Source: CAD feature listing. Evaluate the final solid. Frame: model axes, mm. Face numbers are marked on the shaded views. Give positions to 0.01 mm unless a question says otherwise; leave off trailing zeros. Order: outer loops, then holes, each group sorted by start corner. A loop starts at its lowest first (then second) coordinate and runs counter-clockwise, first axis right, second up.
```python
from build123d import *

# Parameters (mm, degrees)
SKETCH1_W             = 42
SKETCH1_H             = 15.43
BOSS_EXTRUDE1_DEPTH   = 1.5875
F_6_0MM_DOWEL_HOLE1_D = 6


with BuildPart() as part:
    # Sketch1 → Boss-Extrude1 (new body, symmetric)
    with BuildSketch(Plane(origin=(0, 0, 0), x_dir=(1, 0, 0), z_dir=(0, 1, 0))):
        with Locations((21, 7.715)):
            Rectangle(SKETCH1_W, SKETCH1_H)
    extrude(amount=BOSS_EXTRUDE1_DEPTH, both=True)

    # Ø6.0mm Dowel Hole1 (through all)
    with Locations(Plane(origin=(0, 1.5875, 0), x_dir=(1, 0, 0), z_dir=(0, 1, 0))):
        with Locations((37, 5)):
            Hole(F_6_0MM_DOWEL_HOLE1_D / 2)


solid = part.part
```
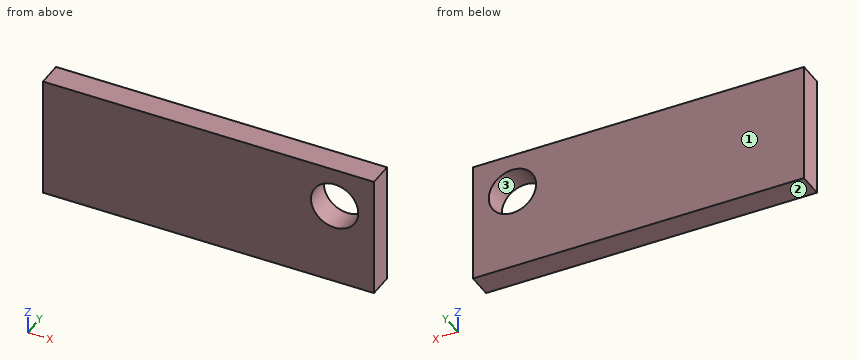
1) Section query B-B, the plane z = -5. Return the cut outline in (x, y), and give its area (3 significant figures).
Report:
outline: (0, -1.59) - (34, -1.59) - (34, 1.59) - (0, 1.59) - close; (40, -1.59) - (42, -1.59) - (42, 1.59) - (40, 1.59) - close
area: 114 mm2
2) Section query C-C, the plane y = -0.9. Return the cut outline in (x, z), and give its area (3 significant figures).
Report:
outline: (0, -15.43) - (42, -15.43) - (42, 0) - (0, 0) - close; hole circle Ø6 at (37, -5)
area: 620 mm2
3) Section query A-A, the plane x = 37. Return the cut outline in (y, z), and give its area (3 significant figures).
Report:
outline: (-1.59, -15.43) - (1.59, -15.43) - (1.59, -8) - (-1.59, -8) - close; (-1.59, -2) - (1.59, -2) - (1.59, 0) - (-1.59, 0) - close
area: 29.9 mm2
4) Draft query along Z for the marked faces 1, 2 and 3. Return one class per face: +Z half, -Z half, draft (parallel to the pull), parting line (faces both ways), or undercut.
Report:
face 1: draft
face 2: -Z half
face 3: undercut
5) Material intervals for L1, parallel to Z at x = 37, y = -0.05; L2, parallel to X at y = 1.1, z = -2.5, sorted ascending.
Report:
L1: z = -15.43 to -8, -2 to 0
L2: x = 0 to 35.34, 38.66 to 42
